Autodesk Inventor part; units mm, degrees
ref_plane "YZ Plane" through (0, 0, 0) normal (1, 0, 0) x (0, 1, 0)
ref_plane "XZ Plane" through (0, 0, 0) normal (0, 1, 0) x (-1, 0, 0)
ref_plane "XY Plane" through (0, 0, 0) normal (0, 0, 1) x (1, 0, 0)
sketch "Sketch1" plane through (0, 0, 0) normal (0, 0, 1) x (1, 0, 0)
  line L0 (10, -7.5) -> (-10, -7.5)
  line L1 (-10, -7.5) -> (-10, 7.5)
  line L2 (-10, 7.5) -> (10, 7.5)
  line L3 (10, 7.5) -> (10, -7.5)
  line L4 (10, -7.5) -> (-10, 7.5) construction
  line L5 (-10, -7.5) -> (10, 7.5) construction
  line L6 (-10, 7.5) -> (10, 7.5)
  line L7 (10, 7.5) -> (10, 13.5)
  line L8 (10, 13.5) -> (-10, 13.5)
  line L9 (-10, 13.5) -> (-10, 7.5)
  line L10 (-10, -7.5) -> (10, -7.5)
  line L11 (10, -7.5) -> (10, -13.5)
  line L12 (10, -13.5) -> (-10, -13.5)
  line L13 (-10, -13.5) -> (-10, -7.5)
  point P0 (0, 0)
  dimension "d0" = 15
  dimension "d1" = 20
  dimension "d2" = 6
extrude "Extrusion1" add sketch "Sketch1" against normal blind 15
extrude "Extrusion2" add sketch "Sketch1" along normal blind 25 contours L11 L12 L13 L0 | L2 L9 L8 L7
sketch "Sketch2" plane through (-10, 13.5, -15) normal (0, 1, 0) x (1, 0, 0)
  line L0 (20, -15) -> (0, -15)
  line L1 (20, -40) -> (0, -40) construction
  line L2 (10, -40) -> (10, -30) construction
  circle A0 centre (10, -30) radius 4
  point P0 (10, -15)
  dimension "d7" = 8
  dimension "d8" = 10
extrude "Extrusion3" cut sketch "Sketch2" against normal through all
fillet "Fillet1" radius 5 4 edges at (-10, 10.5, 25) (10, 10.5, 25) (-10, -10.5, 25) (10, -10.5, 25)
sketch "Sketch3" plane through (0, 0, -15) normal (0, 0, -1) x (-1, 0, 0)
  circle A0 centre (0, 0) radius 2.15
  dimension "d12" = 4.3
extrude "Extrusion4" cut sketch "Sketch3" against normal through all
chamfer "Chamfer1" distance 2 angle 45 6 edges at (8.5355, 13.5, 23.5355) (0, 13.5, 25) (-8.5355, 13.5, 23.5355) (8.5355, -13.5, 23.5355) (0, -13.5, 25) (-8.5355, -13.5, 23.5355)
chamfer "Chamfer2" distance 4 angle 45 1 edges at (-10, 0, 0)
properties part number "cylinder clevis"
Build history of the part. All positions in model axes, mm. A direction names the side the tool comes from. Give positions to 0.01 mm unless a question says otherwise; leave off trailing zeros. Order: outer loops, then holes, each group sorted by start corner. A loop starts at its lowest first (then second) coordinate and runs counter-clockwise, first axis right, second up. Notation, with made-up numbers: M 8,26 L 39,26 A28 ccw 39,53 Z; hole C 83,63.5 d11. An arc over 180 degrees is marked long. Write item = value, one per line. Start each with the question number.
(1) Slice it at D-D on z = 8.5. Write the cut outline in (x, y).
(2) Slice it at C-C on z = 15. Write the cut outline in (x, y), plus the area to 3 significant figures.
(3) Slice it at B-B on y = 10.75. Write the cut outline in (x, z).
(4) Slice it at A-A on x = 0. Write the cut outline in (y, z).
(5) Probe L1, parallel to Z at x = 0, y = 9.5; L2, parallel to Y at x = -7.25, z = 14; L3, parallel to X at y = -8.9, z = 15. List the from-to ranges inside material, lowest first. Write a range as [from, to].
(6) Which spindle directions (+Z, -Z, +X, -X, +Y, -Y) get a long thin tool onto all of the face, cutting with end or side? Do faces 4 (the flat face through (-8, 0, -2)), 5 (the flat face through (0.1, -12.5, 24)), 6 (the flat face through (4, 0, 0)). Say none if no direction does.
(7) Two-plate mould, pull along X, no slides. Class faces 1 (the flat face through (0, -9, 25)), 2 (the cylindrical face through (2.15, 0.09, -7.6)), 3 (the flat face through (10, 0, -1)): released by +X, released by -X, zero draft, split by the parting line, or undercut.
Responses:
q1.outline = M -10,-11.5 L -8,-13.5 L 8,-13.5 L 10,-11.5 L 10,-7.5 L -10,-7.5 Z; M -10,7.5 L 10,7.5 L 10,11.5 L 8,13.5 L -8,13.5 L -10,11.5 Z
q2.outline = M -10,-11.5 L -8,-13.5 L -4,-13.5 L -4,-7.5 L -10,-7.5 Z; M -10,7.5 L -4,7.5 L -4,13.5 L -8,13.5 L -10,11.5 Z; M 4,-13.5 L 8,-13.5 L 10,-11.5 L 10,-7.5 L 4,-7.5 Z; M 4,7.5 L 10,7.5 L 10,11.5 L 8,13.5 L 4,13.5 Z
q2.area = 136 mm2
q3.outline = M -10,-15 L 10,-15 L 10,20 A5 ccw 5,25 L -5,25 A5 ccw -10,20 Z; hole C 0,15 d8
q4.outline = M -13.5,-15 L -2.15,-15 L -2.15,0 L -7.5,0 L -7.5,11 L -13.5,11 Z; M -13.5,19 L -7.5,19 L -7.5,25 L -11.5,25 L -13.5,23 Z; M 2.15,-15 L 13.5,-15 L 13.5,11 L 7.5,11 L 7.5,0 L 2.15,0 Z; M 7.5,19 L 13.5,19 L 13.5,23 L 11.5,25 L 7.5,25 Z
q5.L1 = [-15, 11], [19, 25]
q5.L2 = [-13.5, -7.5], [7.5, 13.5]
q5.L3 = [-10, -4], [4, 10]
q6.face_4 = +Z, -X
q6.face_5 = +Z, +X, -X, -Y
q6.face_6 = +Z, +X, -X
q7.face_1 = zero draft
q7.face_2 = undercut
q7.face_3 = released by +X
